Geometry: final body of the model. Coordinates: model frame, mm. A direction names the side the tool comes from. Give positions to 0.01 mm unless a question says otherwise; leave off trailing zeros. Loops run counter-clockwise (first coordinate to the right, second up) from the corner with the lowest first, then second, coordinate; pieces in that order, holes last. Notation, with made-up numbers: (-31.75, -35.75) - (-15.75, -35.75) arc R14 ccw to (-15.75, -30.75) - close; hole circle Ø8 at (72, 30). An arc over 180 degrees is marked (long way). Answer in a Markdown table with one row per item.
from build123d import *

# Parameters (mm, degrees)
CROQUIS1_R              = 1.65
SALIENTE_EXTRUIR1_DEPTH = 4
CROQUIS2_W              = 30.8
CROQUIS2_H              = 4.2
SALIENTE_EXTRUIR2_DEPTH = 4
CROQUIS3_W              = 8.5
CROQUIS3_H              = 20.5
CORTAR_EXTRUIR1_DEPTH   = 4
REDONDEO1_R             = 4
REDONDEO2_R             = 4
CHAFL_N1_SIZE           = 1
CROQUIS4_R              = 2.8
CORTAR_EXTRUIR2_DEPTH   = 1


with BuildPart() as part:
    # Croquis1 → Saliente-Extruir1 (new body)
    with BuildSketch(Plane(origin=(0, 0, 0), x_dir=(1, 0, 0), z_dir=(0, 1, 0))):
        Polygon((0, 0), (0, 45), (45, 45), (45, 35), (10, 35), (10, 0), align=None)
        with Locations(Location((35, 40, 0), (0, 0, 270))):
            Circle(CROQUIS1_R, mode=Mode.SUBTRACT)
        with Locations(Location((5, 10, 0), (0, 0, 270))):
            Circle(CROQUIS1_R, mode=Mode.SUBTRACT)
    extrude(amount=SALIENTE_EXTRUIR1_DEPTH)

    # Croquis2 → Saliente-Extruir2 (add)
    with BuildSketch(Plane(origin=(0, 4, 0), x_dir=(1, 0, 0), z_dir=(0, 1, 0))):
        with Locations((29.6, 32.9)):
            Rectangle(CROQUIS2_W, CROQUIS2_H)
        Polygon((10, 35), (10, 0), (14.2, 0), (14.2, 30.8), (14.2, 35), align=None)
    extrude(amount=-SALIENTE_EXTRUIR2_DEPTH)

    # Croquis3 → Cortar-Extruir1 (cut)
    with BuildSketch(Plane(origin=(0, 4, 0), x_dir=(1, 0, 0), z_dir=(0, 1, 0))):
        Polygon((29, 45), (0, 45), (0, 36.5), (8.5, 36.5), (29, 36.5), align=None)
        with Locations((4.25, 26.25)):
            Rectangle(CROQUIS3_W, CROQUIS3_H)
    extrude(amount=-CORTAR_EXTRUIR1_DEPTH, mode=Mode.SUBTRACT)

    # Redondeo1
    redondeo1_edges = [part.edges().sort_by_distance(p)[0] for p in [
        (14.2, 2, -30.8),
        (8.5, 2, -36.5),
    ]]
    fillet(redondeo1_edges, radius=REDONDEO1_R)

    # Redondeo2
    redondeo2_edges = [part.edges().sort_by_distance(p)[0] for p in [
        (0, 2, 0),
        (45, 2, -45),
        (0, 2, -16),
        (29, 2, -45),
    ]]
    fillet(redondeo2_edges, radius=REDONDEO2_R)

    # Chaflán1
    chafl_n1_edges = [part.edges().sort_by_distance(p)[0] for p in [
        (31.6, 4, -30.8),
        (14.2, 4, -13.4),
        (15.371572875, 4, -29.628427125),
    ]]
    chamfer(chafl_n1_edges, length=CHAFL_N1_SIZE)

    # Croquis4 → Cortar-Extruir2 (cut)
    with BuildSketch(Plane(origin=(0, 4, 0), x_dir=(1, 0, 0), z_dir=(0, 1, 0))):
        with Locations(Location((35, 40, 0), (0, 0, 270))):
            Circle(CROQUIS4_R)
        with Locations(Location((5, 10, 0), (0, 0, 270))):
            Circle(CROQUIS4_R)
    extrude(amount=-CORTAR_EXTRUIR2_DEPTH, mode=Mode.SUBTRACT)


solid = part.part
Q1. Cut plane A-A (x = 5). Output: boundary loops of the cut face in (y, z).
Check values:
| item | result |
|---|---|
| outline | (0, -16) - (4, -16) - (4, -12.8) - (3, -12.8) - (3, -11.65) - (0, -11.65) - close; (0, -8.35) - (3, -8.35) - (3, -7.2) - (4, -7.2) - (4, 0) - (0, 0) - close |
Q2. Draft query along X for faces 1 (the flat face through (3, 3, -10)), 2 (the flat face through (31, 2, -30.8)), 3 (the flat face through (29, 2, -39)). Return one class per face: pulls with the +X half, pulls with the -X half, needs draft (parallel to the pull), parting line crosses it, or undercut.
Check values:
| item | result |
|---|---|
| face 1 | undercut |
| face 2 | needs draft |
| face 3 | pulls with the -X half |
Q3. Reachability of faces 4 (the flat face through (14.2, 2, -13)), 5 (the cylindrical face through (2.516, 3.507, -8.708)), 6 (the flat face through (6, 2, -16)) from +Z, -Z, +X, -X, +Y, -Y: full face, straight path, thin tool, end or side. Return the list, or none.
Check values:
| item | result |
|---|---|
| face 4 | +Z, +X, +Y, -Y |
| face 5 | +Y |
| face 6 | -Z, -X, +Y, -Y |
Q4. Cut plane B-B (z = -40). Output: boundary loops of the cut face in (x, y), and give its area (3 significant figures).
Check values:
| item | result |
|---|---|
| outline | (29, 0) - (33.35, 0) - (33.35, 3) - (32.2, 3) - (32.2, 4) - (29, 4) - close; (36.65, 0) - (45, 0) - (45, 4) - (37.8, 4) - (37.8, 3) - (36.65, 3) - close |
| area | 48.5 mm² |
Q5. First-contact query: pin 1 (4 mm diameter, centred on x = 35, z = -40, fed in from +Y); pin 2 (2 mm diameter, centred on x = 23.5, y = 2.5, fed in from -Z); pin 3 (1.2 mm diameter, centred on y = 1, z = -39, fed in from -X). Flat tips, straight axial feed; report the tip coordinate or a pass-through.
Check values:
| item | result |
|---|---|
| pin 1 | y = 3 |
| pin 2 | z = -36.5 |
| pin 3 | x = 29 |
Q6. Cut plane D-D (x = 35). Output: boundary loops of the cut face in (y, z).
Check values:
| item | result |
|---|---|
| outline | (0, -45) - (4, -45) - (4, -42.8) - (3, -42.8) - (3, -41.65) - (0, -41.65) - close; (0, -38.35) - (3, -38.35) - (3, -37.2) - (4, -37.2) - (4, -31.8) - (3, -30.8) - (0, -30.8) - close |
Q7. Material intervals for line 1 along Z through (x, y) = (35, 1.8); line 2 along X through (y, z) = (1.75, -10); line 3 along X through (y, z) = (3.4, -40), sorted ascending.
Check values:
| item | result |
|---|---|
| line 1 | -45 to -41.65, -38.35 to -30.8 |
| line 2 | 0 to 3.35, 6.65 to 14.2 |
| line 3 | 29 to 32.2, 37.8 to 45 |
Q8. Cut plane C-C (y = 0.8). Output: boundary loops of the cut face in (x, z).
Check values:
| item | result |
|---|---|
| outline | (0, -12) arc R4 ccw to (4, -16) - (8.5, -16) - (8.5, -32.5) arc R4 ccw to (12.5, -36.5) - (29, -36.5) - (29, -41) arc R4 ccw to (33, -45) - (41, -45) arc R4 ccw to (45, -41) - (45, -30.8) - (18.2, -30.8) arc R4 cw to (14.2, -26.8) - (14.2, 0) - (4, 0) arc R4 ccw to (0, -4) - close; hole circle Ø3.3 at (5, -10); hole circle Ø3.3 at (35, -40) |
